Here's how the part is built. I have some questions about the finished solid (model axes, mm). A direction names the side the tool comes from. Coordinates: 2 decimals unless noted, no trailing zeros. Loops run counter-clockwise (first coordinate to the right, second up) from the corner with the lowest first, then second, coordinate; pieces in that order, holes last. Notation, with made-up numbers: (-18, 36.25) -> (33, 36.25) arc R10 cw to (33, 49.25) -> close; hole circle Ø11 at (-12.75, 46.25). An arc over 180 degrees is marked (long way). Answer as a JSON object with one key per item and string values. Group by question number.
Q1. I need wall thicknesses on line 1 (X direction, y = 3, z = 12.5) (3 decimals); line 2 (X direction, y = -1.5, z = 34.5) (3 decimals); line 3 (Y direction, x = -2.5, z = 19). Which ranges of each line are inside material? Lowest first, please.
Q2. Thinking about a two-plate mould opening in Y: for faces 4 (the cylindrical face through (11.105, 0.156, 12.038)), 5 (the cylindrical face through (14.399, 1.251, 16.767)), 6 (the flat face through (14, -11.112, 22)), which applies, released by +Y, released by -Y, zero draft, split by the parting line, or undercut?
Q3. On a 3-axis mill with a long thin cutter (end or side, diameter ignored), from which of +Z, -Z, +X, -X, +Y, -Y can I reach the whole of each face in a straight line? I mean faces 1 (the flat face through (-6.35, -7, 22)), 2 (the flat face through (9.525, 17, 3)), 3 (the cylindrical face through (14.063, 7.667, 23.938)). Say none if no direction works.
Q4. I want a section at A-A on y = -5. Write out the boundary of the cut face in (x, z) (3 decimals).
Q5. I'm going to push flat-ended pins straight in: pin 1 (5.5 mm diameter, centred on x = 12.7, z = 12.7, fed in from +Y); pin 2 (7 mm diameter, centred on x = -15.88, y = 17.46, fed in from +Z); pin 3 (6.5 mm diameter, centred on x = 1.5, z = 28, fed in from -Y). Where does each tip first touch, or does it pass through?
Q6. I want a section at D-D on y = 16. Write out the boundary of the cut face in (x, z) (3 decimals).
```python
from build123d import *

# Parameters (mm, degrees)
F0_W      = 44.45
F0_H      = 22.225
F1_DEPTH  = 44.45
F2_W      = 12.7
F2_H      = 44.45
F3_DEPTH  = 15.875
F5_W      = 12.7
F5_H      = 6.35
F6_DEPTH  = 12.7
F8_D      = 4.4958
F10_D     = 3.4544
F12_R     = 3.9878
F13_DEPTH = 44.451
F14_R     = 6.15188
F15_DEPTH = 28.575
F17_D     = 3.4544
F17_DEPTH = 12.7
F17_TIP   = 1.0378064612


# Not quite as in the source:
# - an extrude ends at something that could not be found from the text; its depth is read off the source's solid
# - a pattern or mirror of a feature is missing from the dataset's text; its kind, count and spacing are read off the source's solid


with BuildPart() as f1:
    # F0 (on Top) → F1 (new body)
    with BuildSketch(Plane.XY):
        Rectangle(F0_W, F0_H)
    extrude(amount=F1_DEPTH)

    # F2 (on face) → F3 (cut)
    with BuildSketch(Plane.XZ.offset(11.1125)):
        with Locations((0, 22.225)):
            Rectangle(F2_W, F2_H)
    extrude(amount=-F3_DEPTH, mode=Mode.SUBTRACT)

    # F5 (on face) → F6 (join)
    with BuildSketch(Plane(origin=(0, 11.1125, 0), x_dir=(-1, 0, 0), z_dir=(0, 1, 0))):
        with Locations((15.875, 3.175)):
            Rectangle(F5_W, F5_H)
    f6 = extrude(amount=F6_DEPTH)

    # F6_copies: F6 across plane
    add(f6.mirror(Plane(origin=(0, 0, 0), x_dir=(0, 0, 1), z_dir=(1, 0, 0))))

    # F8 (through all)
    with Locations(Plane.XY.offset(6.35)):
        with Locations((-15.875, 17.4625)):
            f8 = Hole(F8_D / 2)

    # F8_copies: F8 across plane
    add(f8.mirror(Plane(origin=(0, 0, 0), x_dir=(0, 0, 1), z_dir=(1, 0, 0))), mode=Mode.SUBTRACT)

    # F10 (through all)
    with Locations(Plane.XZ.offset(11.1125)):
        with Locations((-12.7, 31.75), (12.7, 12.7)):
            Hole(F10_D / 2)

    # F12 (on face) → F13 (cut, through all)
    with BuildSketch(Plane(origin=(-22.225, 0, 0), x_dir=(0, -1, 0), z_dir=(-1, 0, 0))):
        with Locations((1.5875, 22.225)):
            Circle(F12_R)
    extrude(amount=-F13_DEPTH, mode=Mode.SUBTRACT)

    # F14 (on face) → F15 (cut, through all)
    with BuildSketch(Plane.YZ.offset(22.225)):
        with Locations((-1.5875, 22.225)):
            Circle(F14_R)
    extrude(amount=-F15_DEPTH, mode=Mode.SUBTRACT)

    # F17
    with Locations(Plane(origin=(0, 11.1125, 0), x_dir=(-1, 0, 0), z_dir=(0, 1, 0))):
        with Locations((-14.2875, 22.225), (14.2875, 22.225)):
            Hole(F17_D / 2, depth=F17_DEPTH)
            with Locations((0, 0, -(F17_DEPTH + F17_TIP / 2))):  # 118° drill point
                Cone(0, F17_D / 2, F17_TIP, mode=Mode.SUBTRACT)


solid = f1.part
```
Result set:
{
 "1": {"line 1": "x = -22.225 to -6.35, 6.35 to 10.984, 14.416 to 22.225", "line 2": "x = -22.225 to -6.35, 6.35 to 22.225", "line 3": "y = 4.76 to 11.11"},
 "2": {"face 4": "zero draft", "face 5": "undercut", "face 6": "released by -Y"},
 "3": {"face 1": "+Z, -Z, -Y", "face 2": "+Z, -Z, +Y", "face 3": "+Y"},
 "4": {"outline": "(-22.225, 0) -> (-6.35, 0) -> (-6.35, 20.162) -> (-22.225, 20.162) -> close; (-22.225, 24.288) -> (-6.35, 24.288) -> (-6.35, 44.45) -> (-22.225, 44.45) -> close; (6.35, 0) -> (22.225, 0) -> (22.225, 17.106) -> (6.35, 17.106) -> close; (6.35, 27.344) -> (22.225, 27.344) -> (22.225, 44.45) -> (6.35, 44.45) -> close; hole circle Ø3.454 at (-12.7, 31.75); hole circle Ø3.454 at (12.7, 12.7)"},
 "5": {"pin 1": "stops at y = 11.11", "pin 2": "stops at z = 6.35", "pin 3": "stops at y = 4.76"},
 "6": {"outline": "(-22.225, 0) -> (-17.582, 0) -> (-17.582, 6.35) -> (-22.225, 6.35) -> close; (-14.168, 0) -> (-9.525, 0) -> (-9.525, 6.35) -> (-14.168, 6.35) -> close; (9.525, 0) -> (14.168, 0) -> (14.168, 6.35) -> (9.525, 6.35) -> close; (17.582, 0) -> (22.225, 0) -> (22.225, 6.35) -> (17.582, 6.35) -> close"}
}
